from build123d import *

# Parameters (mm, degrees)
F0_R     = 2
F0_W     = 48
F0_H     = 56
F1_DEPTH = 3
F2_W     = 58
F2_H     = 66
F2_W_2   = 54
F2_H_2   = 62
F3_DEPTH = 10
F4_R     = 2
F5_DEPTH = 150
F6_R     = 2
F7_DEPTH = 150


with BuildPart() as f1:
    # F0 (on Top) → F1 (new body)
    with BuildSketch(Plane.XY):
        with BuildLine():
            Line((-29, -33), (29, -33))
            Line((29, -33), (34.187102, -29.978189))
            ThreePointArc((34.187102, -29.978189), (35.641388, -29.315702), (37.198334, -28.955486))
            ThreePointArc((37.198334, -28.955486), (41.977715, -23.994613), (38.164283, -18.257848))
            ThreePointArc((38.164283, -18.257848), (36.059717, -17.229965), (34.343039, -15.636616))
            ThreePointArc((34.343039, -15.636616), (30.753152, -9.568991), (29, -2.740388))
            ThreePointArc((29, -2.740388), (28.849352, 0), (29, 2.740388))
            ThreePointArc((29, 2.740388), (30.753152, 9.568991), (34.343039, 15.636616))
            ThreePointArc((34.343039, 15.636616), (36.059717, 17.229965), (38.164283, 18.257848))
            ThreePointArc((38.164283, 18.257848), (41.989676, 23.836841), (37.510905, 28.906299))
            ThreePointArc((37.510905, 28.906299), (36.345626, 29.216653), (35.240235, 29.698633))
            Line((35.240235, 29.698633), (29, 33))
            Line((29, 33), (-29, 33))
            Line((-29, 33), (-35.523929, 29.622473))
            ThreePointArc((-35.523929, 29.622473), (-36.536989, 29.183773), (-37.600798, 28.888714))
            ThreePointArc((-37.600798, 28.888714), (-41.99229, 23.791117), (-38.164283, 18.257848))
            ThreePointArc((-38.164283, 18.257848), (-36.059717, 17.229965), (-34.343039, 15.636616))
            ThreePointArc((-34.343039, 15.636616), (-30.753152, 9.568991), (-29, 2.740388))
            ThreePointArc((-29, 2.740388), (-28.849352, 0), (-29, -2.740388))
            ThreePointArc((-29, -2.740388), (-30.753152, -9.568991), (-34.343039, -15.636616))
            ThreePointArc((-34.343039, -15.636616), (-36.059717, -17.229965), (-38.164283, -18.257848))
            ThreePointArc((-38.164283, -18.257848), (-41.987222, -23.874692), (-37.436242, -28.919728))
            ThreePointArc((-37.436242, -28.919728), (-36.183275, -29.24235), (-34.998701, -29.76273))
            Line((-34.998701, -29.76273), (-29, -33))
        make_face()
        with Locations((-36.5, -23.5)):
            Circle(F0_R, mode=Mode.SUBTRACT)
        with Locations((36.5, -23.5)):
            Circle(F0_R, mode=Mode.SUBTRACT)
        with Locations((-36.5, 23.5)):
            Circle(F0_R, mode=Mode.SUBTRACT)
        Rectangle(F0_W, F0_H, mode=Mode.SUBTRACT)
        with Locations((36.5, 23.5)):
            Circle(F0_R, mode=Mode.SUBTRACT)
        with BuildLine():
            ThreePointArc((29, 2.740388), (28.849352, 0), (29, -2.740388))
            Line((29, -2.740388), (29, 2.740388))
        make_face()
        with BuildLine():
            Line((-29, 2.740388), (-29, -2.740388))
            ThreePointArc((-29, -2.740388), (-28.849352, 0), (-29, 2.740388))
        make_face()
    extrude(amount=F1_DEPTH)

    # F2 (on face) → F3 (join)
    with BuildSketch(Plane.XY.offset(3)):
        Rectangle(F2_W, F2_H)
        Rectangle(F2_W_2, F2_H_2, mode=Mode.SUBTRACT)
    extrude(amount=F3_DEPTH)

    # F4 (on face) → F5 (cut)
    with BuildSketch(Plane.XZ.offset(33)):
        with Locations((-15, 8)):
            Circle(F4_R)
        with Locations((15, 8)):
            Circle(F4_R)
    extrude(amount=-F5_DEPTH, mode=Mode.SUBTRACT)

    # F6 (on face) → F7 (cut)
    with BuildSketch(Plane.YZ.offset(29)):
        with Locations((-16, 8)):
            Circle(F6_R)
        with Locations((16, 8)):
            Circle(F6_R)
    extrude(amount=-F7_DEPTH, mode=Mode.SUBTRACT)


solid = f1.part
Can you work these out from the model? Positions are in its coordinate system, mm. A direction names the side the tool comes from. Round coordinates to 2 decimals unless told otherwise and drop trailing zeros. Loops run counter-clockwise (first coordinate to the right, second up) from the corner with the lowest first, then second, coordinate; pieces in that order, holes last. Notation, with made-up numbers: (-22, 38.25) - (-1, 38.25) arc R18 ccw to (-1, 72.25) - close; hole circle Ø8 at (79.5, -9). An arc over 180 degrees is marked (long way). Write item = value, one per line. Start each with the question number.
(1) If we section it at C-C (y = -23.5): Please give me the cut outline in (x, z), and give its area (3 significant figures).
(2) If we mould it in two halves opening along Y, with no side actions, what happens to faces 1 (the face through (-30.79, 9.66, 1.48)), 2 (the face through (36.4, 29.2, 1.5)), 3 (the face through (-36.2, -29.236, 1.479))? For each: released by +Y, released by -Y, zero draft, split by the parting line, or undercut.
(3) If we section it at D-D (x = -36.5): Please give me the cut outline in (y, z).
(4) If we section it at B-B (z = 1): Give the number of separate pieces and of enclosed holes in the cut face, and give its area (3 significant figures).
(5) If I drill on probe 1 along X at (y, z) = (18, 8.75); probe 2 along Z at (x, y) = (15, -31.7); probe 3 along Y at (x, z) = (-12, 10), over which ranges is the centre line in solid material (lowest first)? Write a range as [from, to].
(6) If we section it at A-A (x = 0): Please give me the cut outline in (y, z), and give its area (3 significant figures).
(7) For P1, Ø6, axis at y = 25.5, z = 1.5, coming from the -X side; P2, Ø10, axis at x = 6, y = -21, coming from the -Z side; P3, Ø6.5, axis at x = -35, y = -12.5, coming from the +Z side; P4, Ø3.5, axis at y = -6, z = 2, coming from the +X side, each with a flat end and sliding along its axis, tell me the tip position at first contact or that it passes through.
(8) For faces 4 (the face through (36.09, -17.25, 1.48)), 5 (the face through (-34, -21, 3)), 6 (the face through (0, 31, 8)), 7 (the face through (-30.715, -9.477, 1.479)), 8 (the face through (34, -21, 3)), which set-ups out of +Z, -Z, +X, -X, +Y, -Y let a thin tool reach every point of the face, with its end or its side?
Ans:
q1.outline = (-42, 0) - (-38.5, 0) - (-38.5, 3) - (-42, 3) - close; (-34.5, 0) - (-24, 0) - (-24, 3) - (-27, 3) - (-27, 13) - (-29, 13) - (-29, 3) - (-34.5, 3) - close; (24, 0) - (34.5, 0) - (34.5, 3) - (29, 3) - (29, 13) - (27, 13) - (27, 3) - (24, 3) - close; (38.5, 0) - (42, 0) - (42, 3) - (38.5, 3) - close
q1.area = 124 mm²
q2.face_1 = undercut
q2.face_2 = released by +Y
q2.face_3 = released by -Y
q3.outline = (-29.14, 0) - (-25.5, 0) - (-25.5, 3) - (-29.14, 3) - close; (-21.5, 0) - (-17.51, 0) - (-17.51, 3) - (-21.5, 3) - close; (17.51, 0) - (21.5, 0) - (21.5, 3) - (17.51, 3) - close; (25.5, 0) - (29.2, 0) - (29.2, 3) - (25.5, 3) - close
q4.separate_pieces = 1
q4.enclosed_holes = 5
q4.area = 1,830 mm²
q5.probe_1 = [-29, -27], [27, 29]
q5.probe_2 = [0, 6], [10, 13]
q5.probe_3 = [-33, -31], [31, 33]
q6.outline = (-33, 0) - (-28, 0) - (-28, 3) - (-31, 3) - (-31, 13) - (-33, 13) - close; (28, 0) - (33, 0) - (33, 13) - (31, 13) - (31, 3) - (28, 3) - close
q6.area = 70.0 mm²
q7.P1 = -42
q7.P2 = through
q7.P3 = 3
q7.P4 = 30.08
q8.face_4 = +Z, -Z, +X
q8.face_5 = +Z, -X, +Y, -Y
q8.face_6 = +Z
q8.face_7 = +Z, -Z, -X
q8.face_8 = +Z, +X, +Y, -Y
